Design review of the part built by this model. Coordinates are the model's own, in mm. A direction names the side the tool comes from. Round coordinates to 2 decimals unless told otherwise and drop trailing zeros. Loops run counter-clockwise (first coordinate to the right, second up) from the corner with the lowest first, then second, coordinate; pieces in that order, holes last. Notation, with made-up numbers: (16, -19) -> (25, -19) arc R20 cw to (25, -9) -> close; hole circle Ø11 at (51, 58). An arc over 180 degrees is marked (long way). Answer as CSV lines item,"result". Start each with the question number.
```python
from build123d import *

# Parameters (mm, degrees)
ESQUISSE1_W        = 15.5
ESQUISSE1_H        = 19.5
BOSS_EXTRU_1_DEPTH = 16
ESQUISSE2_R        = 0.55
ESQUISSE2_R_2      = 0.3
BOSS_EXTRU_2_DEPTH = 5
BOSS_EXTRU_3_START = 1.6
ESQUISSE4_R        = 1.1
ESQUISSE4_R_2      = 0.8
BOSS_EXTRU_3_DEPTH = 0.05
CONG_1_R           = 0.6


with BuildPart() as part:
    # Esquisse1 → Boss.-Extru.1 (new body)
    with BuildSketch(Plane(origin=(0, 0, 0), x_dir=(1, 0, 0), z_dir=(0, 1, 0))):
        with Locations((7.75, 9.75)):
            Rectangle(ESQUISSE1_W, ESQUISSE1_H)
    extrude(amount=BOSS_EXTRU_1_DEPTH)

    # Esquisse2 → Boss.-Extru.2 (add)
    with BuildSketch(Plane.XZ):
        with Locations(Location((1.75, -3.9, 0), (0, 0, 270))):
            Circle(ESQUISSE2_R)
        with Locations(Location((13.75, -3.9, 0), (0, 0, 270))):
            Circle(ESQUISSE2_R)
        with Locations(Location((7.75, -18.1, 0), (0, 0, 270))):
            Circle(ESQUISSE2_R)
        with Locations(Location((1.75, -16.1, 0), (0, 0, 270))):
            Circle(ESQUISSE2_R_2)
        with Locations(Location((13.75, -16.1, 0), (0, 0, 270))):
            Circle(ESQUISSE2_R_2)
    extrude(amount=BOSS_EXTRU_2_DEPTH)

    # Esquisse4 → Boss.-Extru.3 (add)
    with BuildSketch(Plane.XZ.offset(BOSS_EXTRU_3_START)):
        with Locations(Location((1.75, -3.9, 0), (0, 0, 270))):
            Circle(ESQUISSE4_R)
        with Locations(Location((13.75, -3.9, 0), (0, 0, 270))):
            Circle(ESQUISSE4_R)
        with Locations(Location((7.75, -18.1, 0), (0, 0, 270))):
            Circle(ESQUISSE4_R)
        with Locations(Location((1.75, -16.1, 0), (0, 0, 270))):
            Circle(ESQUISSE4_R_2)
        with Locations(Location((13.75, -16.1, 0), (0, 0, 270))):
            Circle(ESQUISSE4_R_2)
    extrude(amount=BOSS_EXTRU_3_DEPTH)

    # Congé1
    # the kernel refuses this fillet: 0.6 mm, written as the material it adds along each edge
    with BuildSketch(Plane(origin=(1.75, -1.65, -3.9), x_dir=(0, 0, -1), z_dir=(1, 0, 0))) as cong_1_piece_1:
        with BuildLine():
            CenterArc((1.15, -0.597913037), CONG_1_R, 94.780191847, 85.219808153)
            Line((0.55, -0.597913037), (0.538, -0.597913037))
            Line((0.538, -0.597913037), (0.538, 0))
            Line((0.538, 0), (0.55, 0.012))
            ThreePointArc((0.55, 0.012), (0.825, 0.012), (1.099, 0.011958261))
            Line((1.099, 0.011958261), (1.1, 0))
        make_face()
    revolve(axis=Axis((1.75, -1.65, -3.9), (0, 1, 0)))
    with BuildSketch(Plane(origin=(13.75, -1.65, -3.9), x_dir=(0, 0, -1), z_dir=(1, 0, 0))) as cong_1_piece_2:
        with BuildLine():
            CenterArc((1.15, -0.597913037), CONG_1_R, 94.780191847, 85.219808153)
            Line((0.55, -0.597913037), (0.538, -0.597913037))
            Line((0.538, -0.597913037), (0.538, 0))
            Line((0.538, 0), (0.55, 0.012))
            ThreePointArc((0.55, 0.012), (0.825, 0.012), (1.099, 0.011958261))
            Line((1.099, 0.011958261), (1.1, 0))
        make_face()
    revolve(axis=Axis((13.75, -1.65, -3.9), (0, 1, 0)))
    with BuildSketch(Plane(origin=(7.75, -1.65, -18.1), x_dir=(0, 0, -1), z_dir=(1, 0, 0))) as cong_1_piece_3:
        with BuildLine():
            CenterArc((1.15, -0.597913037), CONG_1_R, 94.780191847, 85.219808153)
            Line((0.55, -0.597913037), (0.538, -0.597913037))
            Line((0.538, -0.597913037), (0.538, 0))
            Line((0.538, 0), (0.55, 0.012))
            ThreePointArc((0.55, 0.012), (0.825, 0.012), (1.099, 0.011958261))
            Line((1.099, 0.011958261), (1.1, 0))
        make_face()
    revolve(axis=Axis((7.75, -1.65, -18.1), (0, 1, 0)))
    with BuildSketch(Plane(origin=(1.75, -1.65, -16.1), x_dir=(0, 0, -1), z_dir=(1, 0, 0))) as cong_1_piece_4:
        with BuildLine():
            CenterArc((0.9, -0.591607978), CONG_1_R, 99.594068227, 80.405931773)
            Line((0.3, -0.591607978), (0.288, -0.591607978))
            Line((0.288, -0.591607978), (0.288, 0))
            Line((0.288, 0), (0.3, 0.012))
            ThreePointArc((0.3, 0.012), (0.55, 0.012), (0.798, 0.01183216))
            Line((0.798, 0.01183216), (0.8, 0))
        make_face()
    revolve(axis=Axis((1.75, -1.65, -16.1), (0, 1, 0)))
    with BuildSketch(Plane(origin=(13.75, -1.65, -16.1), x_dir=(0, 0, -1), z_dir=(1, 0, 0))) as cong_1_piece_5:
        with BuildLine():
            CenterArc((0.9, -0.591607978), CONG_1_R, 99.594068227, 80.405931773)
            Line((0.3, -0.591607978), (0.288, -0.591607978))
            Line((0.288, -0.591607978), (0.288, 0))
            Line((0.288, 0), (0.3, 0.012))
            ThreePointArc((0.3, 0.012), (0.55, 0.012), (0.798, 0.01183216))
            Line((0.798, 0.01183216), (0.8, 0))
        make_face()
    revolve(axis=Axis((13.75, -1.65, -16.1), (0, 1, 0)))


solid = part.part
```
Q1. Mouldability with a two-part tool opening along X and no side actions: class faces 1 (the flat face through (13, -1.6, -4)), 2 (the flat face through (2, -5, -4)), 3 (the cylindrical face through (2.21, -0.79, -4.2)), 4 (the flat face through (0, 8, -10)) as pulls with the +X half, pulls with the -X half, needs draft (parallel to the pull), parting line crosses it, or undercut.
Q2. Add section D-D, the plane x = 7.75. Give the boundary of the cut face in (y, z).
Q3. Machinability: for faces 5 (the flat face through (8, 8, -19.5)), 6 (the cylindrical face through (13.213, -3.605, -3.781)), 7 (the cylindrical face through (13.213, -0.789, -3.781)), which of the approach directions +Z, -Z, +X, -X, +Y, -Y give a long, thin tool a straight path to every point of the face, cutting with its end or side? Answer none if there is none.
Q4. Add section C-C, the plane y = -1. Give the boundary of the cut face in (x, z).
Q5. Add section A-A, the plane z = -18.1. Give the boundary of the cut face in (x, y).
Q6. For pin 1 Ø4 at (x, z) = (11.5, -5.5) entering from -Y; pin 2 Ø3 at (x, z) = (5, -11) entering from -Y; pin 3 Ø6 at (y, z) = (4, -2) entering from -X; pin 4 Ø1 at (y, z) = (-2.5, -3.5) entering from +X, all flat-tipped, find the tip position at first contact; note any pin that passes through.
Q7. Add section B-B, the plane x = 13.75. Give the boundary of the cut face in (y, z).
Q8. To check wall thickness, follow probe 1 along Y at (x, z) = (4.25, -15.75); probe 2 along Z at (x, y) = (1.5, -3.25). State the ranges of each line that lie inside material, in increasing order. Write a range as from..to.
Worked answers:
1,face 1,"undercut"
1,face 2,"needs draft"
1,face 3,"undercut"
1,face 4,"pulls with the -X half"
2,outline,"(-5, -18.65) -> (-2.25, -18.65) arc R0.6 cw to (-1.65, -19.2) -> (-1.6, -19.2) -> (-1.6, -18.65) -> (0, -18.65) -> (0, -19.5) -> (16, -19.5) -> (16, 0) -> (0, 0) -> (0, -17.55) -> (-1.6, -17.55) -> (-1.6, -17) -> (-1.65, -17) arc R0.6 cw to (-2.25, -17.55) -> (-5, -17.55) -> close"
3,face 5,"-Z, +X, -X, +Y, -Y"
3,face 6,"-Y"
3,face 7,"none"
4,outline,"circle Ø1.1 at (1.75, -3.9); circle Ø0.6 at (1.75, -16.1); circle Ø1.1 at (7.75, -18.1); circle Ø1.1 at (13.75, -3.9); circle Ø0.6 at (13.75, -16.1)"
5,outline,"(0, 0) -> (7.2, 0) -> (7.2, -1.6) -> (6.65, -1.6) -> (6.65, -1.65) arc R0.6 cw to (7.2, -2.25) -> (7.2, -5) -> (8.3, -5) -> (8.3, -2.25) arc R0.6 cw to (8.85, -1.65) -> (8.85, -1.6) -> (8.3, -1.6) -> (8.3, 0) -> (15.5, 0) -> (15.5, 16) -> (0, 16) -> close"
6,pin 1,"stops at y = -1.79"
6,pin 2,"stops at y = 0"
6,pin 3,"stops at x = 0"
6,pin 4,"stops at x = 14.31"
7,outline,"(-5, -16.4) -> (-2.24, -16.4) arc R0.6 cw to (-1.65, -16.9) -> (-1.6, -16.9) -> (-1.6, -16.4) -> (0, -16.4) -> (0, -19.5) -> (16, -19.5) -> (16, 0) -> (0, 0) -> (0, -3.35) -> (-1.6, -3.35) -> (-1.6, -2.8) -> (-1.65, -2.8) arc R0.6 cw to (-2.25, -3.35) -> (-5, -3.35) -> (-5, -4.45) -> (-2.25, -4.45) arc R0.6 cw to (-1.65, -5) -> (-1.6, -5) -> (-1.6, -4.45) -> (0, -4.45) -> (0, -15.8) -> (-1.6, -15.8) -> (-1.6, -15.3) -> (-1.65, -15.3) arc R0.6 cw to (-2.24, -15.8) -> (-5, -15.8) -> close"
8,probe 1,"y = 0..16"
8,probe 2,"z = -16.27..-15.93, -4.39..-3.41"
